Here's how the part is built. I have some questions about the finished solid (model axes, mm). A direction names the side the tool comes from. Give positions to 0.01 mm unless a question says otherwise; leave off trailing zeros. Loops run counter-clockwise (first coordinate to the right, second up) from the corner with the lowest first, then second, coordinate; pieces in that order, holes last.
Q1. Suppose I cut it at B-B (z = 18). List the corners of the cut face in (x, y) for me.
Q2. I'm going to push flat-ended pins straight in: P1, Ø1, axis at y = 3.5, z = -11, coming from the -X side; P2, Ø0.5, axis at x = 32, y = -2, coming from the +Z side; P3, Ø0.8, axis at x = -45.5, y = 8, coming from the +Z side. Where does each tip first touch, or does it pass through?
Q3. Suppose I cut it at C-C (z = 26). List the corners of the cut face in (x, y) for me, and give its area (3 significant figures).
Q4. Thinking about a two-plate mould opening in X: for faces 1 (the face through (48.274, 0.986, -34.423)), 2 (the face through (-36.839, 3, 15)), 3 (the face through (23, -4, -12)), 4 (the face through (0, 1, -12)), which applies, pulls with the +X half, pulls with the -X half, needs draft (parallel to the pull), parting line crosses it, or undercut?
Q5. For faces 5 (the face through (2.5, -4, -11)), 6 (the face through (-42, 3, -10)), 7 (the face through (-42, 3, 16)), 8 (the face through (-46.839, 3, -11)), 9 (the face through (43.5, -4, -11)), which set-ups out of +Z, -Z, +X, -X, +Y, -Y let a thin tool reach every point of the face, with its end or its side?
Q6. I need wall thicknesses on probe 1 along X at (y, z) = (1.4, -33.5); probe 2 along Z at (x, y) = (39, -5.5); probe 3 along Y at (x, z) = (21, 11). Which ranges of each line are inside material? Lowest first, please.
Q7. Suppose I cut it at D-D (x = -29). List the corners of the cut face in (y, z) for me.
Q8. Suppose I cut it at A-A (z = -33.5). List the corners of the cut face in (x, y) for me, and give its area (3 significant figures).
```python
from build123d import *

# Parameters (mm, degrees)
SKETCH1_W           = 100
SKETCH1_H           = 74
SKETCH1_R           = 2
SKETCH1_R_2         = 1.5
BOSS_EXTRUDE1_DEPTH = 2
SKETCH2_W           = 10
SKETCH2_H           = 2
BOSS_EXTRUDE2_DEPTH = 2
SKETCH3_W           = 41
SKETCH3_H           = 2
SKETCH3_W_2         = 1
SKETCH3_H_2         = 1
BOSS_EXTRUDE4_DEPTH = 8
SKETCH4_W           = 1
SKETCH4_H           = 1
BOSS_EXTRUDE5_DEPTH = 8


with BuildPart() as part:
    # Sketch1 → Boss-Extrude1 (new body)
    with BuildSketch(Plane(origin=(0, 0, 0), x_dir=(1, 0, 0), z_dir=(0, 1, 0))):
        Rectangle(SKETCH1_W, SKETCH1_H)
        with Locations(Location((-46.5, 33.5, 0), (0, 0, 270))):
            Circle(SKETCH1_R, mode=Mode.SUBTRACT)
        with Locations(Location((46.5, 33.5, 0), (0, 0, 90))):
            Circle(SKETCH1_R, mode=Mode.SUBTRACT)
        with Locations(Location((46.5, -33.5, 0), (0, 0, 270))):
            Circle(SKETCH1_R, mode=Mode.SUBTRACT)
        with Locations(Location((-46.5, -33.5, 0), (0, 0, 90))):
            Circle(SKETCH1_R, mode=Mode.SUBTRACT)
        with Locations(Location((46.5, -18, 0), (0, 0, 270))):
            Circle(SKETCH1_R, mode=Mode.SUBTRACT)
        with Locations(Location((45, 15, 0), (0, 0, 270))):
            Circle(SKETCH1_R, mode=Mode.SUBTRACT)
        with Locations(Location((0, 10.5, 0), (0, 0, 270))):
            Circle(SKETCH1_R_2, mode=Mode.SUBTRACT)
        with Locations(Location((46.5, 10.5, 0), (0, 0, 270))):
            Circle(SKETCH1_R_2, mode=Mode.SUBTRACT)
        with Locations(Location((46.5, -13.5, 0), (0, 0, 90))):
            Circle(SKETCH1_R_2, mode=Mode.SUBTRACT)
        with Locations(Location((0, -13.5, 0), (0, 0, 90))):
            Circle(SKETCH1_R_2, mode=Mode.SUBTRACT)
    extrude(amount=BOSS_EXTRUDE1_DEPTH)

    # Sketch2 → Boss-Extrude2 (add)
    with BuildSketch(Plane(origin=(0, 2, 0), x_dir=(1, 0, 0), z_dir=(0, 1, 0))):
        with Locations((-41.839490028, 11)):
            Rectangle(SKETCH2_W, SKETCH2_H)
        with Locations((-41.839490028, -15)):
            Rectangle(SKETCH2_W, SKETCH2_H)
    extrude(amount=BOSS_EXTRUDE2_DEPTH)

    # Sketch3 → Boss-Extrude4 (add)
    # profile 1 of 2: a face of its own
    with BuildSketch(Plane.XZ):
        with Locations((23, 14)):
            Rectangle(SKETCH3_W, SKETCH3_H)
        with Locations((3.5, 14)):
            Rectangle(SKETCH3_W_2, SKETCH3_H_2, mode=Mode.SUBTRACT)
        with Locations((6.0925, 14)):
            Rectangle(SKETCH3_W_2, SKETCH3_H_2, mode=Mode.SUBTRACT)
        with Locations((8.685, 14)):
            Rectangle(SKETCH3_W_2, SKETCH3_H_2, mode=Mode.SUBTRACT)
        with Locations((11.2775, 14)):
            Rectangle(SKETCH3_W_2, SKETCH3_H_2, mode=Mode.SUBTRACT)
        with Locations((13.87, 14)):
            Rectangle(SKETCH3_W_2, SKETCH3_H_2, mode=Mode.SUBTRACT)
        with Locations((16.4625, 14)):
            Rectangle(SKETCH3_W_2, SKETCH3_H_2, mode=Mode.SUBTRACT)
        with Locations((19.055, 14)):
            Rectangle(SKETCH3_W_2, SKETCH3_H_2, mode=Mode.SUBTRACT)
        with Locations((21.6475, 14)):
            Rectangle(SKETCH3_W_2, SKETCH3_H_2, mode=Mode.SUBTRACT)
        with Locations((24.24, 14)):
            Rectangle(SKETCH3_W_2, SKETCH3_H_2, mode=Mode.SUBTRACT)
        with Locations((26.8325, 14)):
            Rectangle(SKETCH3_W_2, SKETCH3_H_2, mode=Mode.SUBTRACT)
        with Locations((29.425, 14)):
            Rectangle(SKETCH3_W_2, SKETCH3_H_2, mode=Mode.SUBTRACT)
        with Locations((32.0175, 14)):
            Rectangle(SKETCH3_W_2, SKETCH3_H_2, mode=Mode.SUBTRACT)
        with Locations((34.61, 14)):
            Rectangle(SKETCH3_W_2, SKETCH3_H_2, mode=Mode.SUBTRACT)
        with Locations((37.2025, 14)):
            Rectangle(SKETCH3_W_2, SKETCH3_H_2, mode=Mode.SUBTRACT)
        with Locations((39.795, 14)):
            Rectangle(SKETCH3_W_2, SKETCH3_H_2, mode=Mode.SUBTRACT)
        with Locations((42.3875, 14)):
            Rectangle(SKETCH3_W_2, SKETCH3_H_2, mode=Mode.SUBTRACT)
    # profile 2 of 2: a face of its own
    with BuildSketch(Plane.XZ):
        with Locations((23, -11)):
            Rectangle(SKETCH3_W, SKETCH3_H)
        with Locations((42.3875, -11)):
            Rectangle(SKETCH3_W_2, SKETCH3_H_2, mode=Mode.SUBTRACT)
        with Locations((39.795, -11)):
            Rectangle(SKETCH3_W_2, SKETCH3_H_2, mode=Mode.SUBTRACT)
        with Locations((37.2025, -11)):
            Rectangle(SKETCH3_W_2, SKETCH3_H_2, mode=Mode.SUBTRACT)
        with Locations((34.61, -11)):
            Rectangle(SKETCH3_W_2, SKETCH3_H_2, mode=Mode.SUBTRACT)
        with Locations((32.0175, -11)):
            Rectangle(SKETCH3_W_2, SKETCH3_H_2, mode=Mode.SUBTRACT)
        with Locations((29.425, -11)):
            Rectangle(SKETCH3_W_2, SKETCH3_H_2, mode=Mode.SUBTRACT)
        with Locations((26.8325, -11)):
            Rectangle(SKETCH3_W_2, SKETCH3_H_2, mode=Mode.SUBTRACT)
        with Locations((24.24, -11)):
            Rectangle(SKETCH3_W_2, SKETCH3_H_2, mode=Mode.SUBTRACT)
        with Locations((21.6475, -11)):
            Rectangle(SKETCH3_W_2, SKETCH3_H_2, mode=Mode.SUBTRACT)
        with Locations((19.055, -11)):
            Rectangle(SKETCH3_W_2, SKETCH3_H_2, mode=Mode.SUBTRACT)
        with Locations((16.4625, -11)):
            Rectangle(SKETCH3_W_2, SKETCH3_H_2, mode=Mode.SUBTRACT)
        with Locations((13.87, -11)):
            Rectangle(SKETCH3_W_2, SKETCH3_H_2, mode=Mode.SUBTRACT)
        with Locations((11.2775, -11)):
            Rectangle(SKETCH3_W_2, SKETCH3_H_2, mode=Mode.SUBTRACT)
        with Locations((8.685, -11)):
            Rectangle(SKETCH3_W_2, SKETCH3_H_2, mode=Mode.SUBTRACT)
        with Locations((6.0925, -11)):
            Rectangle(SKETCH3_W_2, SKETCH3_H_2, mode=Mode.SUBTRACT)
        with Locations((3.5, -11)):
            Rectangle(SKETCH3_W_2, SKETCH3_H_2, mode=Mode.SUBTRACT)
    extrude(amount=BOSS_EXTRUDE4_DEPTH)

    # Sketch4 → Boss-Extrude5 (add)
    with BuildSketch(Plane(origin=(0, 2, 0), x_dir=(1, 0, 0), z_dir=(0, 1, 0))):
        with Locations((-45.839490028, 11)):
            Rectangle(SKETCH4_W, SKETCH4_H)
        with Locations((-43.246990028, 11)):
            Rectangle(SKETCH4_W, SKETCH4_H)
        with Locations((-40.654490028, 11)):
            Rectangle(SKETCH4_W, SKETCH4_H)
        with Locations((-38.061990028, 11)):
            Rectangle(SKETCH4_W, SKETCH4_H)
        with Locations((-38.061990028, -15)):
            Rectangle(SKETCH4_W, SKETCH4_H)
        with Locations((-40.654490028, -15)):
            Rectangle(SKETCH4_W, SKETCH4_H)
        with Locations((-43.246990028, -15)):
            Rectangle(SKETCH4_W, SKETCH4_H)
        with Locations((-45.839490028, -15)):
            Rectangle(SKETCH4_W, SKETCH4_H)
    extrude(amount=BOSS_EXTRUDE5_DEPTH)


solid = part.part
```
Solutions:
1. outline: (-50, 0) - (44.5, 0) - (44.5, 2) - (-50, 2) - close; (48.5, 0) - (50, 0) - (50, 2) - (48.5, 2) - close
2. P1: stops at x = -46.84
2. P2: stops at z = 15
2. P3: stops at z = 15.5
3. outline: (-50, 0) - (50, 0) - (50, 2) - (-50, 2) - close
3. area: 200 mm2
4. face 1: undercut
4. face 2: pulls with the +X half
4. face 3: needs draft
4. face 4: undercut
5. face 5: +Z, -Z, -X, -Y
5. face 6: +X, -X, +Y
5. face 7: +Z, +X, -X, +Y
5. face 8: +Z, -Z, -X, +Y
5. face 9: +Z, -Z, +X, -Y
6. probe 1: x = -50 to -48.5, -44.5 to 44.5, 48.5 to 50
6. probe 2: z = -12 to -10, 13 to 15
6. probe 3: y = 0 to 2
7. outline: (0, -37) - (2, -37) - (2, 37) - (0, 37) - close
8. outline: (-50, 0) - (-48.5, 0) - (-48.5, 2) - (-50, 2) - close; (-44.5, 0) - (44.5, 0) - (44.5, 2) - (-44.5, 2) - close; (48.5, 0) - (50, 0) - (50, 2) - (48.5, 2) - close
8. area: 184 mm2
